```python
from build123d import *

# Parameters (mm, degrees)
BOSS_EXTRUDE3_DEPTH = 50
SKETCH3_R           = 12.5
BOSS_EXTRUDE4_DEPTH = 25
FILLET1_R           = 8


with BuildPart() as part:
    # Sketch1 → Boss-Extrude3 (new body)
    with BuildSketch(Plane.XY):
        Polygon((25, 25), (0, 25), (0, 0), (60, 0), (60, 25), align=None)
        Polygon((0, 0), (0, 25), (-25, 25), (-60, 25), (-60, 0), align=None)
    extrude(amount=BOSS_EXTRUDE3_DEPTH)

    # Sketch3 → Boss-Extrude4 (add)
    with BuildSketch(Plane.XY.offset(50)):
        with BuildLine():
            Line((-25, 75), (-25, 25))
            Line((-25, 25), (25, 25))
            Line((25, 25), (25, 75))
            ThreePointArc((25, 75), (0, 100), (-25, 75))
        make_face()
        with Locations((0, 75)):
            Circle(SKETCH3_R, mode=Mode.SUBTRACT)
    extrude(amount=-BOSS_EXTRUDE4_DEPTH)

    # Fillet1
    fillet1_edges = [part.edges().sort_by_distance(p)[0] for p in [
        (25, 25, 37.5),
        (-25, 25, 37.5),
    ]]
    fillet(fillet1_edges, radius=FILLET1_R)


solid = part.part
```
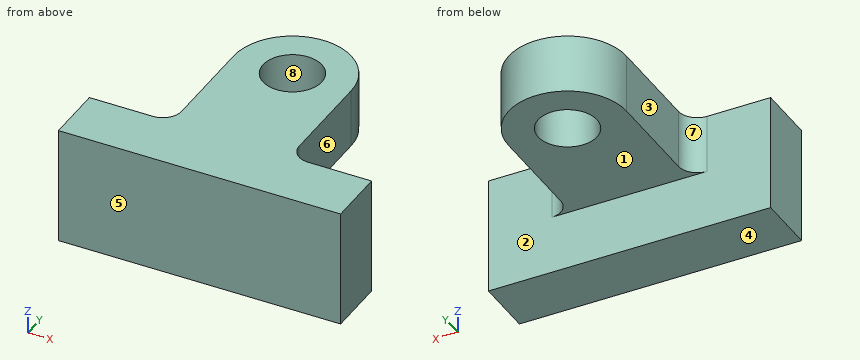
Check sheet for the modelled part. Datum: model origin and axes. Units: mm. Face numbers are marked on the shaded views. A direction names the side the tool comes from. Round coordinates to 2 decimals unless told otherwise and drop trailing zeros. Order: outer loops, then holes, each group sorted by start corner. A loop starts at its lowest first (then second) coordinate and runs counter-clockwise, first axis right, second up. Notation, with made-up numbers: (-7.75, -7) - (27.25, -7) arc R25 cw to (27.25, 20) - close; hole circle Ø1 at (69.25, 72.5). An arc over 180 degrees is marked (long way). Answer as CSV lines item,"result". Start each with the question number.
1) Section check A-A (x = 0). Record the cut outline in (y, z).
2) Section check B-B (y = 64.5). Record the cut outline in (x, z), then the cut area to 3 significant figures.
3) Draft check along X on the marked faces 6, 7 and 8. Enter one of: +X half, -X half, draft (parallel to the pull), parting line (faces both ways), or undercut.
4) Section check C-C (z = 43.5). Record the cut outline in (x, y).
5) Depth check by flat-ended pin: pin 1 (5 mm diameter, centred on y = 63.5, z = 26.5, fed in from -X); pin 2 (4 mm diameter, centred on y = 34.5, z = 42, fed in from +X); pin 3 (6 mm diameter, centred on x = 33.5, z = 41.5, fed in from +Y). Enter the tip coordinate at first touch or a pass-through.
6) Tool access check on the marked faces 1, 2, 3, 4 and 5. Record the directions out of +Z, -Z, +X, -X, +Y, -Y that give a thin tool (end or side, any length) a straight path to the whole face; none if there is none.
7) Scan lines: probe 1 along Y at (x, z) = (0, 35); probe 2 along Z at (x, y) = (-6, 64); probe 3 along Y at (x, z) = (-36, 37). Record each from-to range of solid material in increasing order.
8) Section check D-D (x = -20). Record the cut outline in (y, z), then the cut area to 4 significant figures.
Determined:
1,outline,"(0, 0) - (25, 0) - (25, 25) - (62.5, 25) - (62.5, 50) - (0, 50) - close; (87.5, 25) - (100, 25) - (100, 50) - (87.5, 50) - close"
2,outline,"(-25, 25) - (-6.78, 25) - (-6.78, 50) - (-25, 50) - close; (6.78, 25) - (25, 25) - (25, 50) - (6.78, 50) - close"
2,area,"911 mm^2"
3,face 6,"+X half"
3,face 7,"-X half"
3,face 8,"undercut"
4,outline,"(-60, 0) - (60, 0) - (60, 25) - (33, 25) arc R8 cw to (25, 33) - (25, 75) arc R25 ccw to (-25, 75) - (-25, 33) arc R8 cw to (-33, 25) - (-60, 25) - close; hole circle Ø25 at (0, 75)"
5,pin 1,"x = -25"
5,pin 2,"x = 25.02"
5,pin 3,"y = 25.4"
6,face 1,"-Z, +X, -X, +Y"
6,face 2,"-Z, +Y"
6,face 3,"+Z, -Z, -X, +Y"
6,face 4,"-Z, +X, -X, +Y, -Y"
6,face 5,"+Z, -Z, +X, -X, -Y"
7,probe 1,"0 to 62.5, 87.5 to 100"
7,probe 2,"25 to 50"
7,probe 3,"0 to 25"
8,outline,"(0, 0) - (25, 0) - (25, 25) - (90, 25) - (90, 50) - (0, 50) - close"
8,area,"2,875 mm^2"
